Geometry: see drawing. Coordinates: mm, zero at the bounding-box minimum. A direction names the side the tool comes from. Round coordinates to 2 decimals unless told otherwise and drop trailing zeros. Loops run counter-clockwise (first coordinate to the right, second up) from the corner with the lowest first, then second, coordinate; pieces in that order, holes last. Notation, with made-up numbers: (-22, 19.25) -> (18, 19.25) arc R30 cw to (18, 57.25) -> close; hole circle Ø2 at (-12.5, 72). An arc over 180 degrees is marked (long way). Answer in a Markdown table with one row per item.
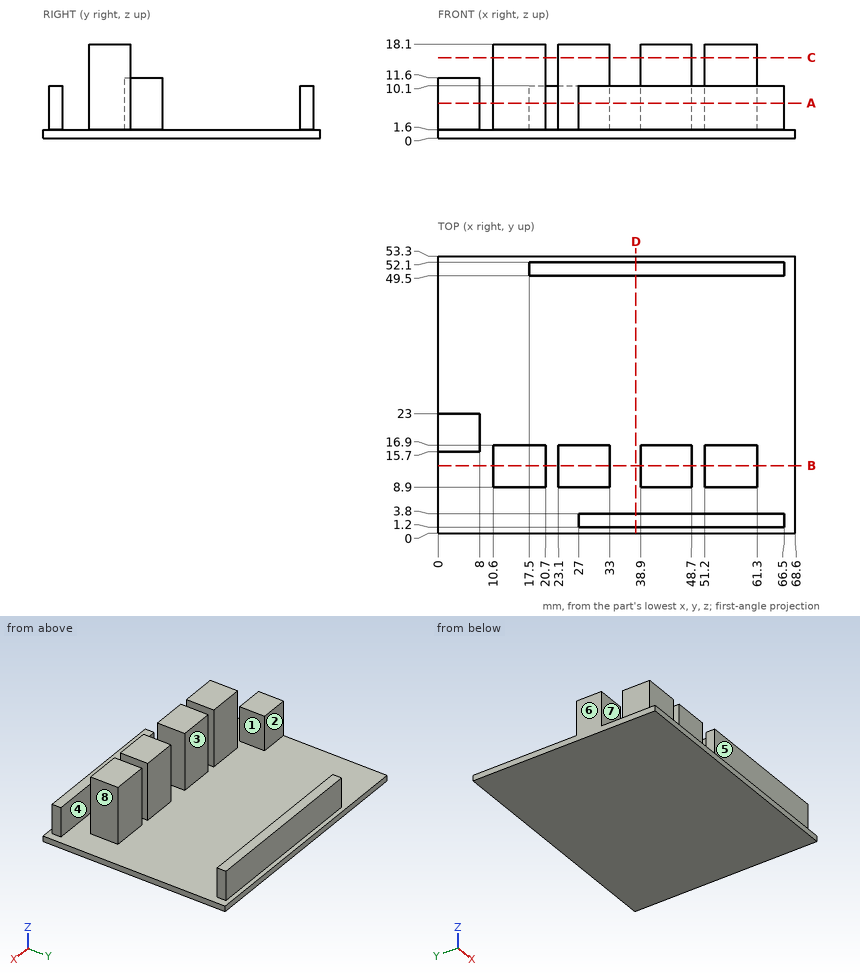
Item 1: Ray query, L1, parallel to X at y = 12, z = 15.5; L2, parallel to Y at x = 27.5, z = 3; L3, parallel to Y at x = 24, z = 5. Return the intervals inside material, ascending.
Ans:
| item | result |
|---|---|
| L1 | 10.6 to 20.7, 23.1 to 33, 38.9 to 48.7, 51.2 to 61.3 |
| L2 | 1.2 to 3.8, 8.9 to 16.9, 49.5 to 52.1 |
| L3 | 8.9 to 16.9, 49.5 to 52.1 |
Item 2: Set-up query: the marked faces 1, 2, 3, 4 and 5. Return all of +Z, -Z, +X, -X, +Y, -Y with unobstructed straight access to the full face (end or side cutting, diameter ignored); none if empty.
Ans:
| item | result |
|---|---|
| face 1 | +Z, +Y, -Y |
| face 2 | +Z, +X, -X, +Y |
| face 3 | +Z, +X |
| face 4 | +Z, +X, -X |
| face 5 | +Z, +X, -X, -Y |
Item 3: Section query B-B, the plane y = 13. Output: boundary loops of the cut face in (x, z).
Ans:
| item | result |
|---|---|
| outline | (0, 0) -> (68.6, 0) -> (68.6, 1.6) -> (61.3, 1.6) -> (61.3, 18.1) -> (51.2, 18.1) -> (51.2, 1.6) -> (48.7, 1.6) -> (48.7, 18.1) -> (38.9, 18.1) -> (38.9, 1.6) -> (33, 1.6) -> (33, 18.1) -> (23.1, 18.1) -> (23.1, 1.6) -> (20.7, 1.6) -> (20.7, 18.1) -> (10.6, 18.1) -> (10.6, 1.6) -> (0, 1.6) -> close |
Item 4: First-contact query: P1, Ø4, axis at y = 12.5, z = 14, coming from the +X side; P2, Ø3, axis at x = 34.5, y = 7.5, coming from the +Z side; P3, Ø1.3, axis at y = 2, z = 4.5, coming from the -X side. Flat tips, straight axial feed; report the tip coordinate or a pass-through.
Ans:
| item | result |
|---|---|
| P1 | x = 61.3 |
| P2 | z = 1.6 |
| P3 | x = 27 |
Item 5: Mould query, pull axis Y, two halves, no side actions, for the marked faces 6, 7 and 8. Classes: released by +Y, released by -Y, zero draft, split by the parting line, or undercut.
Ans:
| item | result |
|---|---|
| face 6 | zero draft |
| face 7 | released by -Y |
| face 8 | undercut |
Item 6: Section query C-C, the plane z = 15.5. Output: boundary loops of the cut face in (x, y).
Ans:
| item | result |
|---|---|
| outline | (10.6, 8.9) -> (20.7, 8.9) -> (20.7, 16.9) -> (10.6, 16.9) -> close; (23.1, 8.9) -> (33, 8.9) -> (33, 16.9) -> (23.1, 16.9) -> close; (38.9, 8.9) -> (48.7, 8.9) -> (48.7, 16.9) -> (38.9, 16.9) -> close; (51.2, 8.9) -> (61.3, 8.9) -> (61.3, 16.9) -> (51.2, 16.9) -> close |
Item 7: Section query D-D, the plane x = 38. Output: boundary loops of the cut face in (y, z), and give its area (3 significant figures).
Ans:
| item | result |
|---|---|
| outline | (0, 0) -> (53.3, 0) -> (53.3, 1.6) -> (52.1, 1.6) -> (52.1, 10.1) -> (49.5, 10.1) -> (49.5, 1.6) -> (3.8, 1.6) -> (3.8, 10.1) -> (1.2, 10.1) -> (1.2, 1.6) -> (0, 1.6) -> close |
| area | 129 mm2 |
Item 8: Section query A-A, the plane z = 6.75. Output: boundary loops of the cut face in (x, y), and give its area (3 significant figures).
Ans:
| item | result |
|---|---|
| outline | (0, 15.7) -> (8, 15.7) -> (8, 23) -> (0, 23) -> close; (10.6, 8.9) -> (20.7, 8.9) -> (20.7, 16.9) -> (10.6, 16.9) -> close; (17.5, 49.5) -> (66.5, 49.5) -> (66.5, 52.1) -> (17.5, 52.1) -> close; (23.1, 8.9) -> (33, 8.9) -> (33, 16.9) -> (23.1, 16.9) -> close; (27, 1.2) -> (66.5, 1.2) -> (66.5, 3.8) -> (27, 3.8) -> close; (38.9, 8.9) -> (48.7, 8.9) -> (48.7, 16.9) -> (38.9, 16.9) -> close; (51.2, 8.9) -> (61.3, 8.9) -> (61.3, 16.9) -> (51.2, 16.9) -> close |
| area | 608 mm2 |
